from build123d import *

# Parameters (mm, degrees)
SKETCH1_W           = 200
SKETCH1_H           = 200
SKETCH1_R           = 10.65
BOSS_EXTRUDE1_DEPTH = 3.75
CUT_EXTRUDE4_START  = -1.5
CUT_EXTRUDE4_DEPTH  = 0.825
CUT_EXTRUDE5_DEPTH  = 3.325
CIRPATTERN1_COUNT   = 4
SKETCH5_W           = 12.1
SKETCH5_H           = 3
CUT_EXTRUDE6_DEPTH  = 10
CIRPATTERN2_COUNT   = 4
SKETCH6_W           = 200
SKETCH6_H           = 200.182674684
SKETCH6_R           = 88.610994186
CUT_EXTRUDE7_DEPTH  = 4.75
SKETCH8_R           = 86.110994186
SKETCH8_R_2         = 84.610994186
BOSS_EXTRUDE2_DEPTH = 13.75
BOSS_EXTRUDE3_DEPTH = 5


with BuildPart() as part:
    # Sketch1 → Boss-Extrude1 (new body)
    with BuildSketch(Plane.XY):
        Rectangle(SKETCH1_W, SKETCH1_H)
        Circle(SKETCH1_R, mode=Mode.SUBTRACT)
    extrude(amount=-BOSS_EXTRUDE1_DEPTH)

    # Sketch2 → Cut-Extrude4 (cut, symmetric)
    with BuildSketch(Plane.XY.offset(CUT_EXTRUDE4_START)):
        with BuildLine():
            Line((8.682868236, 10.918346907), (6.628856395, 8.335512155))
            ThreePointArc((6.628856395, 8.335512155), (3.815515862, 9.943054798), (0.648987911, 10.63020765))
            ThreePointArc((0.648987911, 10.63020765), (0.324644823, 10.645050763), (0, 10.65))
            ThreePointArc((0, 10.65), (-0.324644823, 10.645050763), (-0.648987911, 10.63020765))
            Line((-0.648987911, 10.63020765), (-0.850082756, 13.92407481))
            ThreePointArc((-0.850082756, 13.92407481), (-0.425238994, 13.943517196), (0, 13.95))
            ThreePointArc((0, 13.95), (0.425238994, 13.943517196), (0.850082756, 13.92407481))
            ThreePointArc((0.850082756, 13.92407481), (4.997788382, 13.024001355), (8.682868236, 10.918346907))
        make_face()
    cut_extrude4 = extrude(amount=CUT_EXTRUDE4_DEPTH, both=True, mode=Mode.SUBTRACT)

    # Sketch4 → Cut-Extrude5 (cut, through all)
    with BuildSketch(Plane.XY.offset(-2.325)):
        with BuildLine():
            Line((5.000342926, 9.403141529), (7.076920348, 12.021634597))
            ThreePointArc((7.076920348, 12.021634597), (7.89918002, 11.498063098), (8.682868236, 10.918346907))
            ThreePointArc((8.682868236, 10.918346907), (9.424158272, 10.285316761), (10.119430429, 9.602063726))
            Line((10.119430429, 9.602063726), (8.035757001, 6.989213791))
            ThreePointArc((8.035757001, 6.989213791), (7.363141404, 7.694585672), (6.628856395, 8.335512155))
            ThreePointArc((6.628856395, 8.335512155), (5.839051921, 8.906625212), (5.000342926, 9.403141529))
        make_face()
    cut_extrude5 = extrude(amount=CUT_EXTRUDE5_DEPTH, mode=Mode.SUBTRACT)

    # CirPattern1: Cut-Extrude4, Cut-Extrude5 ×4 about axis
    cirpattern1_axis = Axis((0, 0, 0), (0, 0, 1))
    for i in range(1, CIRPATTERN1_COUNT):
        add(cut_extrude4.rotate(cirpattern1_axis, i * 360 / CIRPATTERN1_COUNT), mode=Mode.SUBTRACT)
        add(cut_extrude5.rotate(cirpattern1_axis, i * 360 / CIRPATTERN1_COUNT), mode=Mode.SUBTRACT)

    # Sketch5 → Cut-Extrude6 (cut)
    with BuildSketch(Plane.XY):
        with Locations((35.9, 23.2)):
            Rectangle(SKETCH5_W, SKETCH5_H)
        with Locations((60.1, 23.2)):
            Rectangle(SKETCH5_W, SKETCH5_H)
        with Locations((11.7, 23.2)):
            Rectangle(SKETCH5_W, SKETCH5_H)
    cut_extrude6 = extrude(amount=-CUT_EXTRUDE6_DEPTH, mode=Mode.SUBTRACT)

    # CirPattern2: Cut-Extrude6 ×4 about axis
    cirpattern2_axis = Axis((0, 0, 0), (0, 0, 1))
    for i in range(1, CIRPATTERN2_COUNT):
        add(cut_extrude6.rotate(cirpattern2_axis, i * 360 / CIRPATTERN2_COUNT), mode=Mode.SUBTRACT)

    # Sketch6 → Cut-Extrude7 (cut, through all)
    with BuildSketch(Plane(origin=(0, 0, -3.75), x_dir=(-1, 0, 0), z_dir=(0, 0, -1))):
        with Locations((0, 0.091337342)):
            Rectangle(SKETCH6_W, SKETCH6_H)
        Circle(SKETCH6_R, mode=Mode.SUBTRACT)
    extrude(amount=-CUT_EXTRUDE7_DEPTH, mode=Mode.SUBTRACT)

    # Sketch8 → Boss-Extrude2 (add)
    with BuildSketch(Plane.XY):
        Circle(SKETCH8_R)
        Circle(SKETCH8_R_2, mode=Mode.SUBTRACT)
        with BuildLine():
            Line((-88.273802601, 7.722957014), (-86.779510554, 7.5922234))
            ThreePointArc((-86.779510554, 7.5922234), (87.110994186, 0), (-86.779510554, -7.5922234))
            Line((-86.779510554, -7.5922234), (-88.273802601, -7.722957014))
            ThreePointArc((-88.273802601, -7.722957014), (88.610994186, 0), (-88.273802601, 7.722957014))
        make_face()
    extrude(amount=-BOSS_EXTRUDE2_DEPTH)

    # Sketch11 → Boss-Extrude3 (add)
    with BuildSketch(Plane.XY):
        with BuildLine():
            Line((76.545964234, -10), (88.044922004, -10))
            ThreePointArc((88.044922004, -10), (87.861366557, -11.501676291), (87.652200718, -13))
            Line((87.652200718, -13), (72.652200718, -13))
            Line((72.652200718, -13), (72.652200718, 13))
            Line((72.652200718, 13), (87.652200718, 13))
            ThreePointArc((87.652200718, 13), (87.861366557, 11.501676291), (88.044922004, 10))
            Line((88.044922004, 10), (76.545964234, 10))
            Line((76.545964234, 10), (76.545964234, -10))
        make_face()
    extrude(amount=BOSS_EXTRUDE3_DEPTH)


solid = part.part
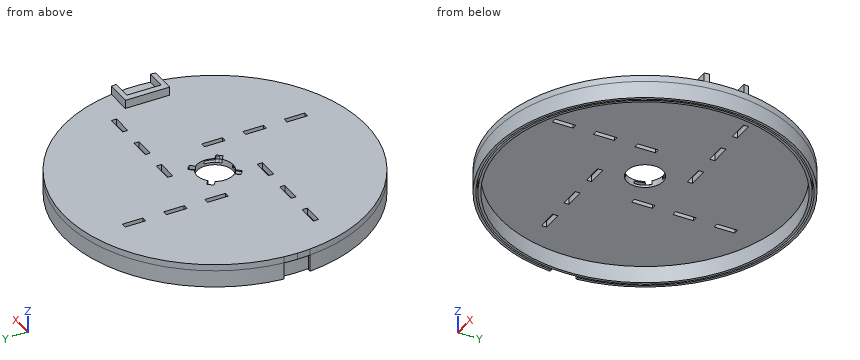
CAD build for the part. Positions are in the model's coordinates, mm. Coordinates: 2 decimals unless noted, no trailing zeros. Order: outer loops, then holes, each group sorted by start corner. A loop starts at its lowest first (then second) coordinate and runs counter-clockwise, first axis right, second up.
Item 1: Band-saw the part on B-B on y = -50. List the corners of the cut face in (x, z), plus the area to 3 significant figures.
Check sheet entries:
outline: (-73.16, -13.75) - (-71.33, -13.75) - (-71.33, -3.75) - (-70.11, -3.75) - (-70.11, -13.75) - (-68.26, -13.75) - (-68.26, -3.75) - (68.26, -3.75) - (68.26, -13.75) - (70.11, -13.75) - (70.11, -3.75) - (71.33, -3.75) - (71.33, -13.75) - (73.16, -13.75) - (73.16, 0) - (-73.16, 0) - close
area: 622 mm2
Item 2: Pin check, flat tips, straight feed: pin 1 Ø2.5 at (x, y) = (-2.5, -11.5) entering from +Z; pin 2 Ø2.5 at (x, z) = (-23.5, -1.5) entering from -Y; pin 3 Ø3 at (x, y) = (0.5, -64) entering from -Z. Stop position of each tip, or through.
Check sheet entries:
pin 1: stops at z = 0
pin 2: stops at y = -85.77
pin 3: stops at z = -3.75
Item 3: Band-saw the part on A-A on z = -7.5. List the corners of the cut face in (x, y).
Check sheet entries:
outline: (-88.27, -7.72) arc R88.61 ccw (long way) to (-88.27, 7.72) - (-86.78, 7.59) arc R87.11 cw (long way) to (-86.78, -7.59) - close; circle Ø172.22 at (0, 0); hole circle Ø169.22 at (0, 0)
Item 4: Drill centre lines: L1, parallel to Y at x = 0, z = -9.25; L2, parallel to X at y = 8.5, z = -12.75; L3, parallel to X at y = -48.5, z = -6.5. Where is each one in solid material? Low to high.
Check sheet entries:
L1: y = -88.61 to -87.11, -86.11 to -84.61, 84.61 to 86.11, 87.11 to 88.61
L2: x = -88.2 to -86.7, -85.69 to -84.18, 84.18 to 85.69, 86.7 to 88.2
L3: x = -74.16 to -72.36, -71.15 to -69.33, 69.33 to 71.15, 72.36 to 74.16
